For this review, use the dimensioned drawing (mm, ordinates from the lowest corner) and the shaded views. A direction names the side the tool comes from. Give positions to 0.01 mm unless a question says otherwise; leave off trailing zeros. Write each loop counter-clockwise with the first axis right and the second up, starting at its lowest first coordinate (ties: lowest second). Pieces come first, ordered by that corner, then holes.
1) Draft analysis for pull direction Y (two halves, no side actions). For the marked faces 3, 4, 5 and 6, state which applies: pulls with the +Y half, pulls with the -Y half, needs draft (parallel to the pull), parting line crosses it, or undercut.
2) We need section C-C on y = 19.05. Give the number of separate pieces and of enclosed holes in the cut face.
3) For P1, Ø9.5, axis at x = 71.5, y = 25.5, coming from the +Z side (3 decimals); P2, Ø9.5, axis at x = 25, y = 24, coming from the +Z side (3 decimals), all flat-tipped, find the tip position at first contact; note any pin that passes through.
4) Wall thickness on line 1 along X through (y, z) = (28, 11) (1 decimal); line 2 along X through (y, z) = (9.5, 27) (3 decimals); line 3 along Y through (x, z) = (19.05, 0.9): over which ranges is each line inside the solid? List them lowest first.
5) We need section B-B on z = 30. Give the boundary of the cut face in (x, y) (3 decimals).
6) Machinability: for the marked faces 1 and 2, which of the approach directions +Z, -Z, +X, -X, +Y, -Y give a long, thin tool a straight path to every point of the face, cutting with its end or side? Answer none if there is none.
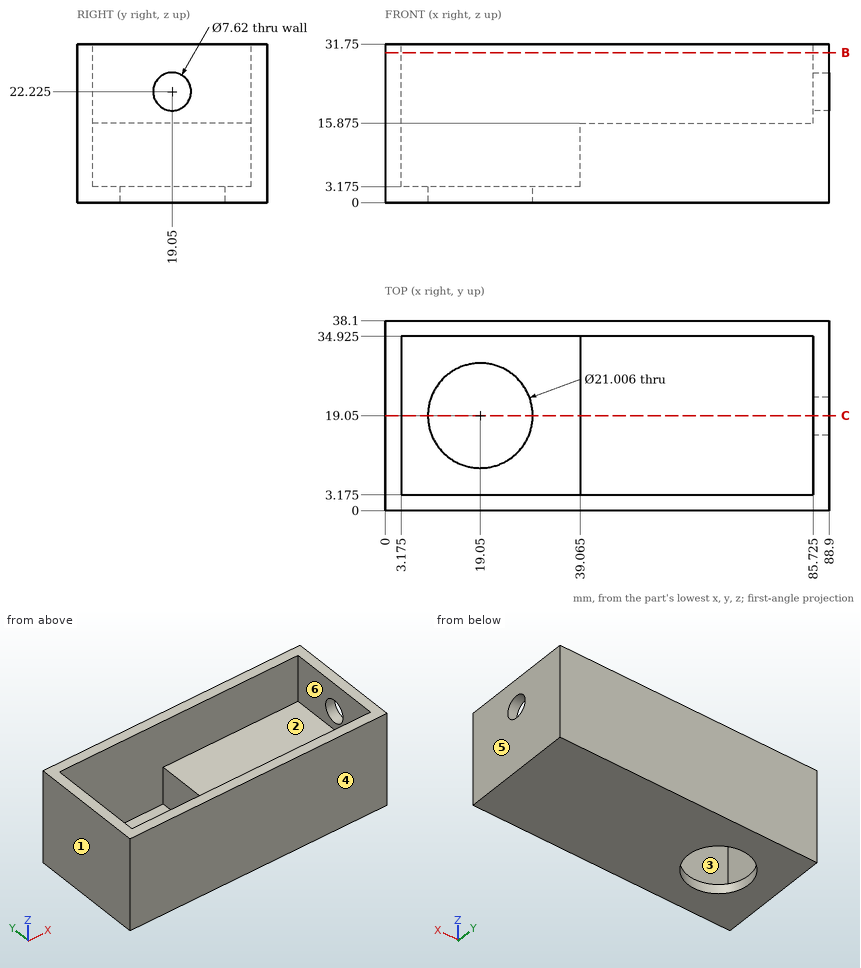
Results list:
1. face 3: undercut
1. face 4: pulls with the -Y half
1. face 5: needs draft
1. face 6: undercut
2. separate pieces: 3
2. enclosed holes: 0
3. P1: stops at z = 15.875
3. P2: stops at z = 3.175
4. line 1: x = 0 to 3.2, 39.1 to 88.9
4. line 2: x = 0 to 3.175, 85.725 to 88.9
4. line 3: y = 0 to 8.55, 29.55 to 38.1
5. outline: (0, 0) - (88.9, 0) - (88.9, 38.1) - (0, 38.1) - close; hole (3.175, 3.175) - (85.725, 3.175) - (85.725, 34.925) - (3.175, 34.925) - close
6. face 1: +Z, -Z, -X, +Y, -Y
6. face 2: +Z
